Source: CAD feature listing. Evaluate the final solid. Frame: model axes, mm. A direction names the side the tool comes from. Round coordinates to 2 decimals unless told otherwise and drop trailing zeros. Order: outer loops, then holes, each group sorted by start corner. A loop starts at its lowest first (then second) coordinate and runs counter-clockwise, first axis right, second up. Notation, with made-up numbers: (56, 58.5) - (82, 58.5) arc R19 ccw to (82, 66.5) - close; hole circle Ø4 at (30, 64). An arc over 180 degrees is marked (long way). Use one line per item in the form item = value. Start each with the question number.
Q1. Set-up query: faces 4 (the cylindrical face through (19.852, 1.972, 12.421)), 5 (the flat face through (0, 6.5, 0)). Return all of +Z, -Z, +X, -X, +Y, -Y with unobstructed straight access to the full face (end or side cutting, diameter ignored); none if empty.
Q2. Cut plane B-B, the plane z = 12.5. Return the cut outline in (x, y), and give its area (3 significant figures).
Q3. Cut plane C-C, the plane y = 2.5. Return the cut outline in (x, z).
Q4. Cut plane A-A, the plane x = 0. Return the cut outline in (y, z), and give its area (3 significant figures).
Q5. Ray query, line 1 (Z direction, x = 0, y = 6.7); line 2 (Z direction, x = 0, y = 5.9); line 3 (X direction, y = 5.8, z = 12.5). Return the intervals inside material, ascending. Write a range as [from, to].
Q6. Cut plane D-D, the plane x = -22. Return the cut outline in (y, z), and give its area (3 significant figures).
Q7. Pin query (flat end, axial travel): pin 1 Ø11 at (x, z) = (0, -25) entering from +Y; pin 2 Ø2 at (x, z) = (-23, 12.5) entering from +Y; pin 3 Ø2 at (y, z) = (5, -20.5) entering from +X; pin 4 Ø3 at (x, y) = (-23, 1.5) entering from -Z. Return the tip coordinate at first contact, or that it passes through.
Q8. Draft query along X for faces 1 (the flat face through (0, 0, 0)), 2 (the cylindrical face through (-29.97, 3.45, -1.32)), 3 (the cylindrical face through (-22.409, 5.521, 15.917)). Return one class per face: released by +X, released by -X, zero draft, split by the parting line, or undercut.
from build123d import *

# Parameters (mm, degrees)
SKETCH1_R           = 30
SKETCH1_R_2         = 1.8
BOSS_EXTRUDE1_DEPTH = 7
SKETCH2_R           = 3.5
CUT_EXTRUDE1_DEPTH  = 3
SKETCH3_R           = 0.75
CUT_EXTRUDE2_DEPTH  = 0.5


with BuildPart() as part:
    # Sketch1 → Boss-Extrude1 (new body)
    with BuildSketch(Plane(origin=(0, 0, 0), x_dir=(1, 0, 0), z_dir=(0, 1, 0))):
        Circle(SKETCH1_R)
        with Locations((0, 25)):
            Circle(SKETCH1_R_2, mode=Mode.SUBTRACT)
        with Locations((21.650635095, -12.5)):
            Circle(SKETCH1_R_2, mode=Mode.SUBTRACT)
        with Locations((-21.650635095, -12.5)):
            Circle(SKETCH1_R_2, mode=Mode.SUBTRACT)
    extrude(amount=BOSS_EXTRUDE1_DEPTH)

    # Sketch2 → Cut-Extrude1 (cut)
    with BuildSketch(Plane(origin=(0, 7, 0), x_dir=(1, 0, 0), z_dir=(0, 1, 0))):
        with Locations((0, 25)):
            Circle(SKETCH2_R)
        with Locations((21.650635095, -12.5)):
            Circle(SKETCH2_R)
        with Locations((-21.650635095, -12.5)):
            Circle(SKETCH2_R)
    extrude(amount=-CUT_EXTRUDE1_DEPTH, mode=Mode.SUBTRACT)

    # Sketch3 → Cut-Extrude2 (cut)
    with BuildSketch(Plane(origin=(0, 7, 0), x_dir=(1, 0, 0), z_dir=(0, 1, 0))):
        Circle(SKETCH3_R)
    extrude(amount=-CUT_EXTRUDE2_DEPTH, mode=Mode.SUBTRACT)


solid = part.part
Completed:
q1.face_4 = +Y, -Y
q1.face_5 = +Y
q2.outline = (-27.27, 0) - (-23.45, 0) - (-23.45, 4) - (-25.15, 4) - (-25.15, 7) - (-27.27, 7) - close; (-19.85, 0) - (19.85, 0) - (19.85, 4) - (18.15, 4) - (18.15, 7) - (-18.15, 7) - (-18.15, 4) - (-19.85, 4) - close; (23.45, 0) - (27.27, 0) - (27.27, 7) - (25.15, 7) - (25.15, 4) - (23.45, 4) - close
q2.area = 311 mm2
q3.outline = circle Ø60 at (0, 0); hole circle Ø3.6 at (-21.65, 12.5); hole circle Ø3.6 at (0, -25); hole circle Ø3.6 at (21.65, 12.5)
q4.outline = (0, -30) - (7, -30) - (7, -28.5) - (4, -28.5) - (4, -26.8) - (0, -26.8) - close; (0, -23.2) - (4, -23.2) - (4, -21.5) - (7, -21.5) - (7, -0.75) - (6.5, -0.75) - (6.5, 0.75) - (7, 0.75) - (7, 30) - (0, 30) - close
q4.area = 384 mm2
q5.line_1 = [-30, -28.5], [-21.5, -0.75], [0.75, 30]
q5.line_2 = [-30, -28.5], [-21.5, 30]
q5.line_3 = [-27.27, -25.15], [-18.15, 18.15], [25.15, 27.27]
q6.outline = (0, -20.4) - (7, -20.4) - (7, 9.02) - (4, 9.02) - (4, 10.73) - (0, 10.73) - close; (0, 14.27) - (4, 14.27) - (4, 15.98) - (7, 15.98) - (7, 20.4) - (0, 20.4) - close
q6.area = 251 mm2
q7.pin_1 = 7
q7.pin_2 = 4
q7.pin_3 = 22.8
q7.pin_4 = -20.92
q8.face_1 = zero draft
q8.face_2 = split by the parting line
q8.face_3 = undercut
